Autodesk Inventor part; units mm, degrees
ref_plane "YZ Plane" through (0, 0, 0) normal (1, 0, 0) x (0, 1, 0)
ref_plane "XZ Plane" through (0, 0, 0) normal (0, 1, 0) x (-1, 0, 0)
ref_plane "XY Plane" through (0, 0, 0) normal (0, 0, 1) x (1, 0, 0)
sketch "Sketch1" plane through (0, 0, 0) normal (0, 1, 0) x (-1, 0, 0)
  line L0 (-4.5709, 0.1557) -> (-12.5709, 0.1557)
  line L1 (-12.5709, 0.1557) -> (-12.5709, 1.3557)
  line L2 (-12.5709, 1.3557) -> (-4.5709, 1.3557)
  line L3 (-4.5709, 1.3557) -> (-4.5709, 0.1557)
  dimension "d27" = 8
  dimension "d28" = 1.3
extrude "Plate4" add sketch "Sketch1" along normal blind 0.25
sketch "Sketch5" plane through (12.3209, 0.25, 1.3557) normal (1, 0, 0) x (0, 1, 0)
  line L0 (0, -1.2) -> (0, 0)
  line L1 (0, 0) -> (-5.7, 0)
  line L2 (-5.7, 0) -> (-5.7, -1.2)
  line L3 (-5.7, -1.2) -> (0, -1.2)
edge flange "Flange4" height 5.7 angle 90 thickness 0.25 bend radius 0.25 thickness toward (1, 0, 0) relief tear relief width 0.25 relief depth 0.125 corner gap 0.25 corner form 0 edges at (12.5709, 0, 0.7557) (4.5709, 0, 0.7557) wall of the first edge with corners at (12.3209, 0.25, 0.1557) (12.3209, 0.25, 1.3557) (12.3209, -5.45, 1.3557) (12.3209, -5.45, 0.1557)
bend "Bend4"
corner "Corner4"
sketch "Sketch6" plane through (12.5709, -5.45, 1.3557) normal (1, 0, 0) x (0, 0, -1)
  line L0 (1.2, 0) -> (0, 0)
  line L1 (0.6, 0) -> (0.6, 5.2) construction
  line L2 (1.2, 5.2) -> (0, 5.2)
  line L3 (1.2, 3.4021) -> (0.85, 3.2)
  line L4 (0.85, 3.2) -> (0.85, 0)
  line L5 (1.2, 0) -> (0.85, 0)
  line L6 (1.2, 5.2) -> (1.2, 0)
  line L7 (1.2, 3.4021) -> (1.2, 0)
  line L8 (0, 5.7) -> (1.2, 5.7)
  point P0 (1.3557, 5.45)
  dimension "d52" = 3.2
  dimension "d54" = 0.25
  dimension "d56" = 2.5
extrude "Cut1" cut sketch "Sketch6" against normal blind 0.25
ref_plane "Work Plane1" through (12.5709, -0.25, 0.7557) normal (0, 0, -1) x (-1, 0, 0)
ref_plane "Work Plane2" through (8.5709, -5.45, 1.3557) normal (1, 0, 0) x (0, 0, -1)
mirror "Mirror1" about plane through (12.5709, -0.25, 0.7557) normal (0, 0, -1) of "Cut1"
mirror "Mirror2" about plane through (8.5709, -5.45, 1.3557) normal (1, 0, 0) of "Cut1"
mirror "Mirror3" about plane through (8.5709, -5.45, 1.3557) normal (1, 0, 0) of "Cut1", "Mirror1"
equation "\"d27\" = atmegaPinBaseWidth"
equation "\"d28\" = atmegaPinWidth1"
equation "\"d52\" = atmegaSeatingPlaneDistance"
equation "\"d54\" = 0.5 * atmegaPinWidth2"
equation "\"d50\" = Thickness"
equation "\"d29\" = Thickness"
equation "\"d40\" = BendReliefWidth"
equation "\"d41\" = BendReliefDepth"
equation "\"d42\" = MinimumRemnant"
equation "\"d43\" = TransitionRadius"
equation "\"d44\" = atmegaPinLenght"
equation "\"d46\" = BendRadius"
equation "\"d47\" = CornerReliefSize"
equation "\"d48\" = GapSize"
equation "\"d49\" = JacobiRadiusSize"
equation "\"BendRadius\" = Thickness"
equation "\"BendReliefWidth\" = Thickness"
equation "\"BendReliefDepth\" = 0.5 * Thickness"
equation "\"CornerReliefSize\" = 4 * Thickness"
equation "\"MinimumRemnant\" = 2 * Thickness"
equation "\"TransitionRadius\" = BendRadius"
equation "\"JacobiRadiusSize\" = BendRadius"
equation "\"GapSize\" = Thickness"
equation "\"atmegaPinThickness\" = 0.3"
equation "\"atmegaPinWidth1\" = 1.3"
equation "\"atmegaPinWidth2\" = 0.5"
equation "\"atmegaEndPinWidth\" = 0.9"
equation "\"atmegaPinBendAngle\" = 80deg"
equation "\"atmegaPinBaseWidth\" = 8"
equation "\"atmegaSeatingPlaneDistance\" = 3.2"
properties part number "atmega_pin"
Geometry check sheet. Reference: the model listing, model coordinates, mm. Give positions to 0.01 mm unless a question says otherwise; leave off trailing zeros. Order: outer loops, then holes, each group sorted by start corner. A loop starts at its lowest first (then second) coordinate and runs counter-clockwise, first axis right, second up.
1. Release check for a two-part mould opening along X. For faces 1 (the face through (12.571, -2, 1)), 2 (the face through (4.571, -2, 1)), 3 (the face through (9, 0.25, 1)), 4 (the face through (4.821, -2, 1)) record: pulls with the +X half, pulls with the -X half, needs draft (parallel to the pull), parting line crosses it, or undercut.
2. Section check A-A, the plane y = -4.1. Enter the section's corners in (x, z), and give its area (3 significant figures).
3. Section check D-D, the plane y = -1.65. Enter the section's corners in (x, z), and give its area (3 significant figures).
4. Section check B-B, the plane z = 0.7. Enter the section's corners in (x, y).
5. Thickness scan on L1, parallel to X at y = -1.2, z = 1.2; L2, parallel to Y at x = 7, z = 0.5; L3, parallel to X at y = -0.1, z = 0.35. Record the ranges inside material, lowest first.
6. Section check C-C, the plane x = 6.5. Enter the section's corners in (y, z).
Values follow:
1. face 1: pulls with the +X half
1. face 2: pulls with the -X half
1. face 3: needs draft
1. face 4: undercut
2. outline: (4.57, 0.51) - (4.82, 0.51) - (4.82, 1.01) - (4.57, 1.01) - close; (12.32, 0.51) - (12.57, 0.51) - (12.57, 1.01) - (12.32, 1.01) - close
2. area: 0.250 mm2
3. outline: (4.57, 0.16) - (4.82, 0.16) - (4.82, 1.36) - (4.57, 1.36) - close; (12.32, 0.16) - (12.57, 0.16) - (12.57, 1.36) - (12.32, 1.36) - close
3. area: 0.600 mm2
4. outline: (4.57, -5.45) - (4.82, -5.45) - (4.82, -0.25) arc R0.25 cw to (5.07, 0) - (12.07, 0) arc R0.25 cw to (12.32, -0.25) - (12.32, -5.45) - (12.57, -5.45) - (12.57, -0.25) arc R0.5 ccw to (12.07, 0.25) - (5.07, 0.25) arc R0.5 ccw to (4.57, -0.25) - close
5. L1: x = 4.57 to 4.82, 12.32 to 12.57
5. L2: y = 0 to 0.25
5. L3: x = 4.59 to 4.87, 12.27 to 12.55
6. outline: (0, 0.16) - (0.25, 0.16) - (0.25, 1.36) - (0, 1.36) - close
